```python
from build123d import *

# Parameters (mm, degrees)
M3_CLEARANCE_HOLE1_D = 3.4
CUT_EXTRUDE1_DEPTH   = 3
CIRPATTERN1_COUNT    = 6
FILLET2_R            = 0.4
CHAMFER1_SIZE        = 0.4


with BuildPart() as part:
    # Sketch5 → Revolve1 (revolve)
    with BuildSketch(Plane.XY, mode=Mode.PRIVATE) as revolve1_sk:
        Polygon((22.1, 0), (30, 0), (30, 5.6), (21.7, 5.6), (21.7, 5.2), (22.1, 4.8), align=None)
    revolve(revolve1_sk.sketch.rotate(Axis((0, 14.134935251, 0), (0, -1, 0)), 180), axis=Axis((0, 14.134935251, 0), (0, -1, 0)))

    # M3 Clearance Hole1 (through all)
    with Locations(Plane(origin=(0, 5.6, 0), x_dir=(1, 0, 0), z_dir=(0, 1, 0))):
        with Locations((27, 0)):
            m3_clearance_hole1 = Hole(M3_CLEARANCE_HOLE1_D / 2)

    # Sketch4 → Cut-Extrude1 (cut)
    with BuildSketch(Plane(origin=(0, 5.6, 0), x_dir=(1, 0, 0), z_dir=(0, 1, 0))):
        with BuildLine():
            Line((27, 3), (29.849623113, 3))
            ThreePointArc((29.849623113, 3), (30, 0), (29.849623113, -3))
            Line((29.849623113, -3), (27, -3))
            ThreePointArc((27, -3), (24, 0), (27, 3))
        make_face()
    cut_extrude1 = extrude(amount=-CUT_EXTRUDE1_DEPTH, mode=Mode.SUBTRACT)

    # CirPattern1: M3 Clearance Hole1, Cut-Extrude1 ×6 about axis
    cirpattern1_axis = Axis((0, 0, 0), (0, 1, 0))
    add([m3_clearance_hole1.rotate(cirpattern1_axis, i * 360 / CIRPATTERN1_COUNT) for i in range(1, CIRPATTERN1_COUNT)], mode=Mode.SUBTRACT)
    add([cut_extrude1.rotate(cirpattern1_axis, i * 360 / CIRPATTERN1_COUNT) for i in range(1, CIRPATTERN1_COUNT)], mode=Mode.SUBTRACT)

    # Fillet2
    fillet2_edges = [part.edges().sort_by_distance(p)[0] for p in [
        (-29.849623113, 4.1, 3),
        (-29.849623113, 4.1, -3),
        (-17.522887768, 4.1, -24.350531909),
        (-12.326735345, 4.1, -27.350531909),
        (12.326735345, 4.1, -27.350531909),
        (17.522887768, 4.1, -24.350531909),
        (29.849623113, 4.1, -3),
        (29.849623113, 4.1, 3),
        (17.522887768, 4.1, 24.350531909),
        (12.326735345, 4.1, 27.350531909),
        (-12.326735345, 4.1, 27.350531909),
        (-17.522887768, 4.1, 24.350531909),
    ]]
    fillet(fillet2_edges, radius=FILLET2_R)

    # Chamfer1
    chamfer1_edges = [part.edges().sort_by_distance(p)[0] for p in [
        (-24, 5.6, 0),
        (-28.202040675, 5.6, -3),
        (-12, 5.6, -20.784609691),
        (-11.502944126, 5.6, -25.923683663),
        (12, 5.6, -20.784609691),
        (16.699096549, 5.6, -22.923683663),
        (-11.502944126, 5.6, 25.923683663),
        (16.699096549, 5.6, 22.923683663),
        (25.980762114, 5.6, 15),
        (28.202040675, 5.6, -3),
        (25.980762114, 5.6, -15),
        (11.502944126, 5.6, -25.923683663),
        (0, 5.6, -30),
        (-16.699096549, 5.6, -22.923683663),
        (-25.980762114, 5.6, -15),
        (-28.202040675, 5.6, 3),
        (-25.980762114, 5.6, 15),
        (0, 5.6, 30),
        (17.565397878, 5.6, 24.156367596),
        (12.137329062, 5.6, 27.290264588),
        (29.702726941, 5.6, 3.133896992),
        (29.702726941, 5.6, -3.133896992),
        (17.565397878, 5.6, -24.156367596),
        (12.137329062, 5.6, -27.290264588),
        (-12.137329062, 5.6, -27.290264588),
        (-17.565397878, 5.6, -24.156367596),
        (-29.702726941, 5.6, -3.133896992),
        (-29.702726941, 5.6, 3.133896992),
        (-17.565397878, 5.6, 24.156367596),
        (-12.137329062, 5.6, 27.290264588),
        (24, 5.6, 0),
        (28.202040675, 5.6, 3),
        (12, 5.6, 20.784609691),
        (11.502944126, 5.6, 25.923683663),
        (-12, 5.6, 20.784609691),
        (-16.699096549, 5.6, 22.923683663),
    ]]
    chamfer(chamfer1_edges, length=CHAMFER1_SIZE - 0.0001)  # a hair under: the kernel refuses the full size


solid = part.part
```
CAD build for the part. Positions are in the model's coordinates, mm. A direction names the side the tool comes from. Round coordinates to 2 decimals unless told otherwise and drop trailing zeros. Loops run counter-clockwise (first coordinate to the right, second up) from the corner with the lowest first, then second, coordinate; pieces in that order, holes last. Notation, with made-up numbers: M -15,31.25 L 44,31.25 A17 cw 44,52.25 Z; hole C 76.5,79.25 d3. An arc over 180 degrees is marked long. Use a Markdown table: item, result. Add a question column.
(1) Flat gauge pins, fed straight in: pin 1 (2 mm diameter, centred on x = 15.5, z = -24.5, fed in from +Y); pin 2 (2.5 mm diameter, centred on x = 28.5, y = 4, fed in from +Z); pin 3 (2.5 mm diameter, centred on x = 28.5, y = 3.5, fed in from -Z). Where does each tip first touch, or does it go through?
(2) Cut at A-A (x = 0). Give the cut face in (y, z), and give its area (3 significant figures).
(3) Cut at C-C (y = 0.85). Give the cut face in (x, z), and give its area (3 significant figures).
(4) Which spindle directions (+Z, -Z, +X, -X, +Y, -Y) get a long thin tool onto all of the face, cutting with end or side? Do faces 1 (the face through (-27.712, 2.636, 11.49)), 2 (the face through (-29, 2.6, 0)), 3 (the face through (24, 4, 0)), 4 (the face through (-11.94, 3.92, -20.82)), 5 (the face through (-16.69, 3.92, -22.91)). Say none if no direction does.
(5) Cut at D-D (x = -13.5). State how many separate pieces and enclosed holes the cut face has, and give its area (3 significant figures).
(6) Cut at B-B (z = 0). Give the cut face in (x, y).
(7) Drill centre lines: line 1 (Z direction, x = 0, y = 3.05); line 2 (Z direction, x = -14, y = 2.2); line 3 (X direction, y = 4.9, z = 23). Where is each one in solid material? Low to high.
(8) Pull direction X, two halves, no side cores. Call faces 6 (the face through (-23.89, 5.31, -0.07)), 7 (the face through (-16.861, 5.397, -22.811)), 8 (the face through (11.511, 3.918, 25.938)), 9 (the face through (13.28, 1.28, 25.07)): +X half, -X half, draft (parallel to the pull), parting line (faces both ways), or undercut.
Geometry says:
| question | item | result |
|---|---|---|
| 1 | pin 1 | stops at y = 2.6 |
| 1 | pin 2 | stops at z = 12.55 |
| 1 | pin 3 | stops at z = -12.55 |
| 2 | outline | M 0,-30 L 5.2,-30 L 5.6,-29.6 L 5.6,-21.7 L 5.2,-21.7 L 4.8,-22.1 L 0,-22.1 Z; M 0,22.1 L 4.8,22.1 L 5.2,21.7 L 5.6,21.7 L 5.6,29.6 L 5.2,30 L 0,30 Z |
| 2 | area | 88.8 mm² |
| 3 | outline | C 0,0 d60; hole C -27,0 d3.4; hole C 0,0 d44.2; hole C -13.5,-23.38 d3.4; hole C -13.5,23.38 d3.4; hole C 13.5,-23.38 d3.4; hole C 13.5,23.38 d3.4; hole C 27,0 d3.4 |
| 3 | area | 1,240 mm² |
| 4 | face 1 | +Y, -Y |
| 4 | face 2 | -X, +Y |
| 4 | face 3 | +X, +Y |
| 4 | face 4 | +Y |
| 4 | face 5 | -Z, +Y |
| 5 | separate pieces | 4 |
| 5 | enclosed holes | 0 |
| 5 | area | 48.4 mm² |
| 6 | outline | M -30,0 L -28.7,0 L -28.7,2.6 L -30,2.6 Z; M -25.3,0 L -22.1,0 L -22.1,4.8 L -21.7,5.2 L -21.7,5.6 L -23.6,5.6 L -24,5.2 L -24,2.6 L -25.3,2.6 Z; M 21.7,5.2 L 22.1,4.8 L 22.1,0 L 25.3,0 L 25.3,2.6 L 24,2.6 L 24,5.2 L 23.6,5.6 L 21.7,5.6 Z; M 28.7,0 L 30,0 L 30,2.6 L 28.7,2.6 Z |
| 7 | line 1 | z = -30 to -22.1, 22.1 to 30 |
| 7 | line 2 | z = -26.53 to -25.01, -21.76 to -17.1, 17.1 to 21.76, 25.01 to 26.53 |
| 7 | line 3 | x = -19.26 to -16.74, -10.52 to 10.52, 16.74 to 19.26 |
| 8 | face 6 | -X half |
| 8 | face 7 | undercut |
| 8 | face 8 | +X half |
| 8 | face 9 | undercut |
